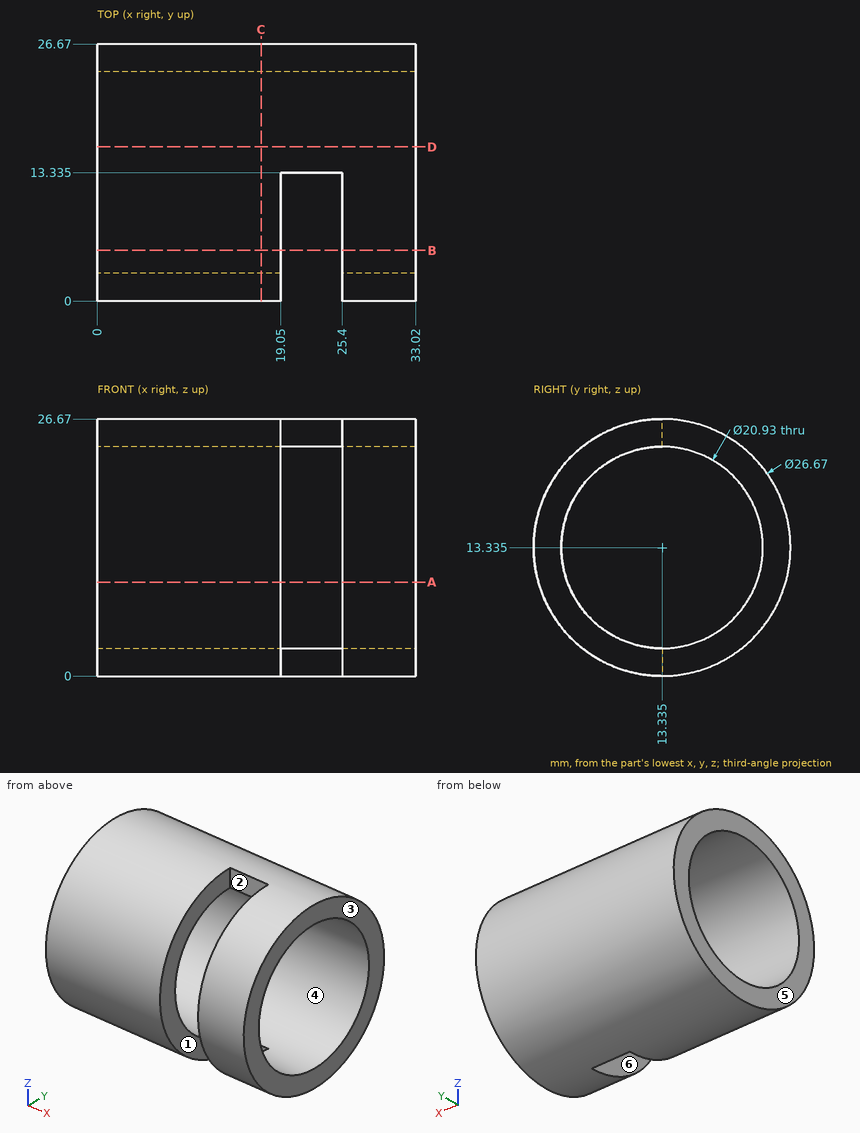
Geometry check sheet. Reference: drawing and pictorial views, mm from the part's lowest x, y, z. A direction names the side the tool comes from. Give positions to 0.01 mm unless a question says otherwise; leave off trailing zeros. Order: outer loops, then holes, each group sorted by start corner. A loop starts at its lowest first (then second) coordinate and runs counter-clockwise, first axis right, second up. Notation, with made-up numbers: M 59.5,22.5 L 102.5,22.5 A29 ccw 102.5,48.5 Z; hole C 4.25,16.25 d1. An arc over 180 degrees is marked long. Answer as a JSON object with one key per item and string values. Group by question number.
1) Cross-section at D-D (y = 16). Enter the section's corners in (x, z) (1 decimal).
2) Cross-section at B-B (y = 5.25). Enter the section's corners in (x, z).
3) Access from +Z, -Z, +X, -X, +Y, -Y to the whole of each face (thin tool, end or side, straight path). Record for the marked faces 5 and 6.
4) Cross-section at A-A (z = 9.75). Enter the section's corners in (x, y), then the cut area to 3 significant figures.
5) Depth check by flat-ended pin: pin 1 Ø2.5 at (x, z) = (22, 25) entering from -Y (3 decimals); pin 2 Ø4 at (x, y) = (17.5, 21) entering from +Z; pin 3 Ø2 at (x, y) = (21.5, 21) entering from +Z (1 decimal). Enter the tip coordinate at first touch or a pass-through.
6) Mould release check, pull along X, two halves, no side actions. Record for the marked faces 1, 2, 3 and 4: released by +X, released by -X, zero draft, split by the parting line, or undercut.
7) Cross-section at C-C (x = 17). Enter the section's corners in (y, z) (1 decimal).
8) Scan lines: line 1 along X through (y, z) = (4.5, 23); line 2 along Y through (x, z) = (29, 18.25) (1 decimal); line 3 along Z through (x, y) = (6.5, 3.75) (1 decimal). Record each from-to range of solid material in increasing order. Write a range as [from, to].
Result sheet:
{
 "1": {"outline": "M 0,0.3 L 33,0.3 L 33,3.2 L 0,3.2 Z; M 0,23.5 L 33,23.5 L 33,26.4 L 0,26.4 Z"},
 "2": {"outline": "M 0,2.73 L 19.05,2.73 L 19.05,6.69 L 0,6.69 Z; M 0,19.98 L 19.05,19.98 L 19.05,23.94 L 0,23.94 Z; M 25.4,2.73 L 33.02,2.73 L 33.02,6.69 L 25.4,6.69 Z; M 25.4,19.98 L 33.02,19.98 L 33.02,23.94 L 25.4,23.94 Z"},
 "3": {"face 5": "+Z, -Z, -X, +Y, -Y", "face 6": "+Z, -Z, -Y"},
 "4": {"outline": "M 0,0.49 L 19.05,0.49 L 19.05,3.5 L 0,3.5 Z; M 0,23.17 L 33.02,23.17 L 33.02,26.18 L 0,26.18 Z; M 25.4,0.49 L 33.02,0.49 L 33.02,3.5 L 25.4,3.5 Z", "area": "180 mm2"},
 "5": {"pin 1": "stops at y = 13.335", "pin 2": "stops at z = 25.41", "pin 3": "stops at z = 24.9"},
 "6": {"face 1": "undercut", "face 2": "undercut", "face 3": "released by +X", "face 4": "zero draft"},
 "7": {"outline": "C 13.3,13.3 d26.7; hole C 13.3,13.3 d20.9"},
 "8": {"line 1": "x = [0, 19.05], [25.4, 33.02]", "line 2": "y = [0.9, 4.1], [22.6, 25.7]", "line 3": "z = [4.1, 9.1], [17.5, 22.6]"}
}
